from build123d import *

# Parameters (mm, degrees)
F0_W           = 75
F0_H           = 82
F1_DEPTH       = 20
F3_D           = 46
F4_D           = 5.5
F4_CBORE_D     = 9.4
F4_CBORE_DEPTH = 6.3
F5_SIZE        = 5


with BuildPart() as f1:
    # F0 (on Front) → F1 (new body)
    with BuildSketch(Plane.XZ):
        Rectangle(F0_W, F0_H)
    extrude(amount=F1_DEPTH)

    # F3 (through all)
    with Locations(Plane.XZ.offset(20)):
        with Locations((0, 0)):
            Hole(F3_D / 2)

    # F4 (through all)
    with Locations(Plane.XZ.offset(20)):
        with Locations((-30, 30), (30, 30)):
            CounterBoreHole(F4_D / 2, F4_CBORE_D / 2, F4_CBORE_DEPTH)

    # F5
    f5_edges = [f1.edges().sort_by_distance(p)[0] for p in [
        (0, -20, -41),
    ]]
    chamfer(f5_edges, length=F5_SIZE)


solid = f1.part
Can you work these out from the model? Positions are in its coordinate system, mm. A direction names the side the tool comes from. Give positions to 0.01 mm unless a question says otherwise; leave off trailing zeros. Loops run counter-clockwise (first coordinate to the right, second up) from the corner with the lowest first, then second, coordinate; pieces in that order, holes last. Notation, with made-up numbers: (22, 54) - (49, 54) arc R5 ccw to (49, 61) - close; hole circle Ø11 at (50.5, 66.25). An arc over 180 degrees is marked (long way). One line per item, written item: value.
(1) I'm going to push flat-ended pins straight in: pin 1 (12 mm diameter, centred on x = -30, z = 30, fed in from +Y); pin 2 (3.5 mm diameter, centred on x = 30, z = 30, fed in from +Y); pin 3 (9 mm diameter, centred on x = -30, z = 30, fed in from -Y). Where does each tip first touch, or does it pass through?
Verdict:
pin 1: y = 0
pin 2: through
pin 3: y = -13.7
(2) If we section it at A-A, the plane x = 30: List the corners of the cut face in (y, z) for me, plus the area to 3 significant figures.
Verdict:
outline: (-20, -36) - (-15, -41) - (0, -41) - (0, 27.25) - (-13.7, 27.25) - (-13.7, 25.3) - (-20, 25.3) - close; (-20, 34.7) - (-13.7, 34.7) - (-13.7, 32.75) - (0, 32.75) - (0, 41) - (-20, 41) - close
area: 1,490 mm^2
(3) If we section it at D-D, the plane y = -11: List the corners of the cut face in (x, z) for me, plus the area to 3 significant figures.
Verdict:
outline: (-37.5, -41) - (37.5, -41) - (37.5, 41) - (-37.5, 41) - close; hole circle Ø5.5 at (-30, 30); hole circle Ø46 at (0, 0); hole circle Ø5.5 at (30, 30)
area: 4,440 mm^2
(4) If we section it at B-B, the plane y = -16.5: List the corners of the cut face in (x, z) for me.
Verdict:
outline: (-37.5, -39.5) - (37.5, -39.5) - (37.5, 41) - (-37.5, 41) - close; hole circle Ø9.4 at (-30, 30); hole circle Ø46 at (0, 0); hole circle Ø9.4 at (30, 30)
(5) On a 3-axis mill with a long thin cutter (end or side, diameter ignored), from which of +Z, -Z, +X, -X, +Y, -Y can I reach the whole of each face in a straight line? I mean faces 5 (the face through (33, -13.7, 30)), 6 (the face through (16, 0, 19)). Say none if no direction works.
Verdict:
face 5: -Y
face 6: +Z, -Z, +X, -X, +Y
(6) If we mould it in two halves opening along X, with no side actions, what happens to faces 1 (the face through (-37.5, -10, -1)), 2 (the face through (-1, -18, -38)), 3 (the face through (37.5, -10, -1)), 4 (the face through (-30, -13.7, 27))? For each: released by +X, released by -X, zero draft, split by the parting line, or undercut.
Verdict:
face 1: released by -X
face 2: zero draft
face 3: released by +X
face 4: undercut
(7) I need wall thicknesses on line 1 along Z through (x, y) = (30, -8.5); line 2 along Z through (x, y) = (-30, -15); line 3 along X through (y, z) = (-4.25, -11). Which ranges of each line are inside material? Lowest first, please.
Verdict:
line 1: -41 to 27.25, 32.75 to 41
line 2: -41 to 25.3, 34.7 to 41
line 3: -37.5 to -20.2, 20.2 to 37.5
(8) If we section it at C-C, the plane z = 0: List the corners of the cut face in (x, y) for me.
Verdict:
outline: (-37.5, -20) - (-23, -20) - (-23, 0) - (-37.5, 0) - close; (23, -20) - (37.5, -20) - (37.5, 0) - (23, 0) - close
